from build123d import *

# Parameters (mm, degrees)
F0_R     = 17.78
F0_R_2   = 6.35
F1_DEPTH = 50.8
F2_DEPTH = 55.245
F3_DEPTH = 67.945
F4_DEPTH = 59.055
F6_D     = 3.3
F6_DEPTH = 7
F6_TIP   = 0.9914200214


with BuildPart() as f1:
    # F0 (on Top) → F1 (new body)
    with BuildSketch(Plane.XY):
        Circle(F0_R)
        Circle(F0_R_2, mode=Mode.SUBTRACT)
    extrude(amount=F1_DEPTH)

    # F0 (on Top) → F2 (join)
    with BuildSketch(Plane.XY):
        Circle(F0_R_2)
        with BuildLine():
            ThreePointArc((0.9525, 1.27), (1.4199031657, 0.7099515829), (1.5875, 0))
            ThreePointArc((1.5875, 0), (1.4199031657, -0.7099515829), (0.9525, -1.27))
            ThreePointArc((0.9525, -1.27), (-1.5875, 0), (0.9525, 1.27))
        make_face(mode=Mode.SUBTRACT)
    extrude(amount=F2_DEPTH)

    # F0 (on Top) → F3 (join)
    with BuildSketch(Plane.XY):
        with BuildLine():
            Line((0.9525, -1.27), (0.9525, 1.27))
            ThreePointArc((0.9525, 1.27), (-1.5875, 0), (0.9525, -1.27))
        make_face()
    extrude(amount=F3_DEPTH)

    # F0 (on Top) → F4 (join)
    with BuildSketch(Plane.XY):
        with BuildLine():
            ThreePointArc((0.9525, -1.27), (1.4199031657, -0.7099515829), (1.5875, 0))
            ThreePointArc((1.5875, 0), (1.4199031657, 0.7099515829), (0.9525, 1.27))
            Line((0.9525, 1.27), (0.9525, -1.27))
        make_face()
    extrude(amount=F4_DEPTH)

    # F6
    with Locations(Plane.XY.offset(50.8)):
        with Locations((0, 12.3825), (0, -12.3825)):
            Hole(F6_D / 2, depth=F6_DEPTH)
            with Locations((0, 0, -(F6_DEPTH + F6_TIP / 2))):  # 118° drill point
                Cone(0, F6_D / 2, F6_TIP, mode=Mode.SUBTRACT)


solid = f1.part
Source: CAD feature listing. Evaluate the final solid. Frame: model axes, mm. A direction names the side the tool comes from. Give positions to 0.01 mm unless a question says otherwise; leave off trailing zeros. Order: outer loops, then holes, each group sorted by start corner. A loop starts at its lowest first (then second) coordinate and runs counter-clockwise, first axis right, second up. Notation, with made-up numbers: (-17.5, 63.5) -> (41.5, 63.5) arc R16 ccw to (41.5, 86.5) -> close; hole circle Ø4 at (25.25, 11). An arc over 180 degrees is marked (long way). Use a Markdown table: item, result.
1) Contact query for flat-ended pins moving along their axis: P1, Ø1, axis at x = 6.5, y = 5, coming from the +Z side; P2, Ø8, axis at y = 12, z = 50.5, coming from the +X side; P3, Ø2.5, axis at x = 0, y = 12.38, coming from the +Z side. Output: stop coordinate, or through.
Answer list:
| item | result |
|---|---|
| P1 | z = 50.8 |
| P2 | x = 15.88 |
| P3 | z = 43.56 |
2) Section query A-A, the plane z = 32. Return the cut outline in (x, y), then the cut area to 3 significant figures.
Answer list:
| item | result |
|---|---|
| outline | circle Ø35.56 at (0, 0) |
| area | 993 mm² |
3) Section query B-B, the plane y = -3.5. Return the cut outline in (x, z) (3 decimals), then the cut area to 3 significant figures.
Answer list:
| item | result |
|---|---|
| outline | (-17.432, 0) -> (17.432, 0) -> (17.432, 50.8) -> (5.298, 50.8) -> (5.298, 55.245) -> (-5.298, 55.245) -> (-5.298, 50.8) -> (-17.432, 50.8) -> close |
| area | 1,820 mm² |
4) Mould query, pull axis Y, two halves, no side actions, for faces 1 (the cylindrical face through (-1.38, -6.2, 52.99)), 2 (the cylindrical face through (0.215, -10.747, 47.251)), 3 (the flat face through (0, -8, 50.8)). Classes: +Y half, -Y half, draft (parallel to the pull), parting line (faces both ways), or undercut.
Answer list:
| item | result |
|---|---|
| face 1 | parting line |
| face 2 | undercut |
| face 3 | draft |
5) Section query C-C, the plane z = 61.5. Return the cut outline in (x, y) (1 decimal).
Answer list:
| item | result |
|---|---|
| outline | (1, -1.3) -> (1, 1.3) arc R1.6 ccw (long way) to start |
6) Reachability of faces 4 (the cylindrical face through (-3.85, -17.36, 25.04)), 5 (the flat face through (1.3, -1.3, 55.245)), 6 (the flat face through (0.952, 0, 63)) from +Z, -Z, +X, -X, +Y, -Y: full face, straight path, thin tool, end or side. Return the list, or none.
Answer list:
| item | result |
|---|---|
| face 4 | +Z, -Z |
| face 5 | +Z |
| face 6 | +Z, +X, +Y, -Y |
7) Section query D-D, the plane x = 10.5. Return the cut outline in (y, z).
Answer list:
| item | result |
|---|---|
| outline | (-14.35, 0) -> (14.35, 0) -> (14.35, 50.8) -> (-14.35, 50.8) -> close |
8) Ray query, line 1 along Y through (x, z) = (0, 46.5); line 2 along Z through (x, y) = (2.5, -4) (3 decimals); line 3 along Z through (x, y) = (11, -0.5). Return the intervals inside material, ascending. Write a range as [from, to].
Answer list:
| item | result |
|---|---|
| line 1 | [-17.78, -14.03], [-10.73, 10.73], [14.03, 17.78] |
| line 2 | [0, 55.245] |
| line 3 | [0, 50.8] |
